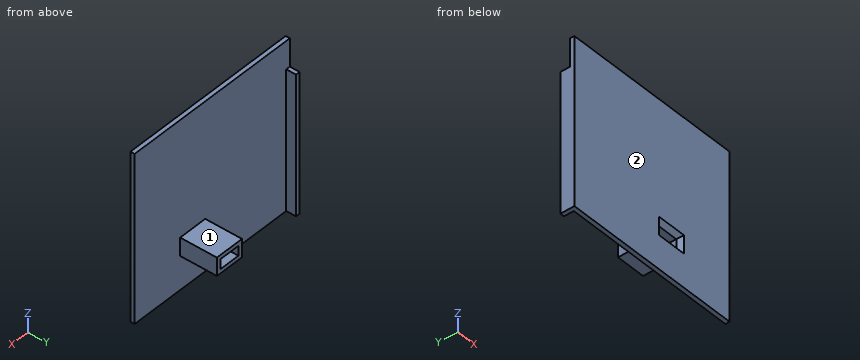
Solid Edge part; units mm, degrees
sketch "Sketch1" plane through (0, 0, 0) normal (0, -1, 0) x (1, 0, 0)
  line L0 (130, 0) -> (130, 120)
  line L1 (130, 120) -> (0, 120)
  line L2 (0, 120) -> (0, 0)
  line L3 (0, 0) -> (130, 0)
extrude "Protrusion1" add sketch "Sketch1" against normal blind 3
sketch "Sketch2" plane through (66.405, 0, 60) normal (0, -1, 0) x (1, 0, 0)
  line L0 (22.4375, -32.9583) -> (7.4375, -32.9583)
  line L1 (7.4375, -32.9583) -> (7.4375, -25.9583)
  line L2 (7.4375, -25.9583) -> (22.4375, -25.9583)
  line L3 (22.4375, -25.9583) -> (22.4375, -32.9583)
extrude "Recorte_Extrudado_3" cut sketch "Sketch2" against normal blind 36.068
chamfer "Chanfro_1" distance 3 angle 45 4 edges at (81.3425, 0, 34.0417) (88.8425, 0, 30.5417) (81.3425, 0, 27.0417) (73.8425, 0, 30.5417)
sketch "Sketch3" plane through (67.905, 3, 60) normal (0, 1, 0) x (-1, 0, 0)
  line L0 (-2.9375, -35.9583) -> (-23.9375, -35.9583)
  line L1 (-23.9375, -35.9583) -> (-23.9375, -22.9583)
  line L2 (-23.9375, -22.9583) -> (-2.9375, -22.9583)
  line L3 (-2.9375, -22.9583) -> (-2.9375, -35.9583)
  line L4 (-5.9375, -32.9583) -> (-20.9375, -32.9583)
  line L5 (-20.9375, -32.9583) -> (-20.9375, -25.9583)
  line L6 (-20.9375, -25.9583) -> (-5.9375, -25.9583)
  line L7 (-5.9375, -25.9583) -> (-5.9375, -32.9583)
extrude "Protrusão_Extrudada_4" add sketch "Sketch3" along normal blind 26.3165
sketch "Sketch4" plane through (66.405, 3, 60) normal (0, 1, 0) x (-1, 0, 0)
  line L0 (66.405, -60) -> (66.405, 40)
  line L1 (66.405, 40) -> (63.405, 40)
  line L2 (63.405, 40) -> (63.405, -60)
  line L3 (63.405, -60) -> (66.405, -60)
extrude "Protrusão_Extrudada_6" add sketch "Sketch4" along normal blind 7
Build history of the part. All positions in model axes, mm. Face numbers are marked on the shaded views. A direction names the side the tool comes from. Coordinates: 2 decimals unless noted, no trailing zeros. Write each loop counter-clockwise with the first axis right and the second up, starting at its lowest first coordinate (ties: lowest second). Pieces come first, ordered by that corner, then holes.
1. Drop flat-ended pins along their axis: pin 1 (10 mm diameter, centred on x = 109.5, z = 76.5, fed in from -Y); pin 2 (2 mm diameter, centred on x = 78.5, z = 18.5, fed in from +Y); pin 3 (1 mm diameter, centred on x = 78, y = 10, fed in from -Z); pin 4 (7.5 mm diameter, centred on x = 79, y = 19, fed in from +Z). Give the stop position or say it passes through.
Answer block:
pin 1: stops at y = 0
pin 2: stops at y = 3
pin 3: stops at z = 24.04
pin 4: stops at z = 37.04
2. Band-saw the part on C-C, the plane y = 27.5. Give the cut face in (x, z), and give its area (3 significant figures).
Answer block:
outline: (70.84, 24.04) - (91.84, 24.04) - (91.84, 37.04) - (70.84, 37.04) - close; hole (73.84, 27.04) - (88.84, 27.04) - (88.84, 34.04) - (73.84, 34.04) - close
area: 168 mm2
3. Drill centre lines: probe 1 along Y at (x, z) = (20.5, 51.5); probe 2 along Z at (x, y) = (90, 10.5); probe 3 along X at (y, z) = (8, 35). Where is each one in solid material? Low to high.
Answer block:
probe 1: y = 0 to 3
probe 2: z = 24.04 to 37.04
probe 3: x = 0 to 3, 70.84 to 91.84
4. Band-saw the part on D-D, the plane z = 22. Give the cut face in (x, y), and give its area (3 significant figures).
Answer block:
outline: (0, 0) - (130, 0) - (130, 3) - (3, 3) - (3, 10) - (0, 10) - close
area: 411 mm2
5. Band-saw the part on A-A, the plane y = 4.75. Give the cut face in (x, z).
Answer block:
outline: (0, 0) - (3, 0) - (3, 100) - (0, 100) - close; (70.84, 24.04) - (91.84, 24.04) - (91.84, 37.04) - (70.84, 37.04) - close; hole (73.84, 27.04) - (88.84, 27.04) - (88.84, 34.04) - (73.84, 34.04) - close
6. 3-axis set-ups, long thin cutter, end or side, ignore diameter. For the marked faces 1 and 2: which of +Z, -Z, +X, -X, +Y, -Y reach the whole face in a straight line?
Answer block:
face 1: +Z, +X, +Y
face 2: +Z, -Z, +X, -X, -Y
7. Band-saw the part on B-B, the plane x = 81. Give the cut face in (y, z), and give its area (3 significant figures).
Answer block:
outline: (0, 0) - (3, 0) - (3, 24.04) - (29.32, 24.04) - (29.32, 27.04) - (3, 27.04) - (0, 24.04) - close; (0, 37.04) - (3, 34.04) - (29.32, 34.04) - (29.32, 37.04) - (3, 37.04) - (3, 120) - (0, 120) - close
area: 488 mm2
